```python
from build123d import *

# Parameters (mm, degrees)
F0_W     = 30
F0_H     = 30
F1_DEPTH = 10
F3_DEPTH = 25


with BuildPart() as f1:
    # F0 (on Front) → F1 (new body)
    with BuildSketch(Plane.XZ):
        with Locations((15, -15)):
            Rectangle(F0_W, F0_H)
    extrude(amount=F1_DEPTH)

    # F2 (on face) → F3 (cut)
    with BuildSketch(Plane.XZ.offset(10)):
        with BuildLine():
            ThreePointArc((5.35, -25), (4, -23.65), (2.65, -25))
            Line((2.65, -25), (5.35, -25))
        make_face()
        with BuildLine():
            Line((5.35, -25), (2.65, -25))
            ThreePointArc((2.65, -25), (4, -26.35), (5.35, -25))
        make_face()
        with BuildLine():
            ThreePointArc((27.35, -25), (26, -23.65), (24.65, -25))
            Line((24.65, -25), (27.35, -25))
        make_face()
        with BuildLine():
            Line((27.35, -25), (24.65, -25))
            ThreePointArc((24.65, -25), (26, -26.35), (27.35, -25))
        make_face()
        with BuildLine():
            Line((27.35, -5), (24.65, -5))
            ThreePointArc((24.65, -5), (26, -6.35), (27.35, -5))
        make_face()
        with BuildLine():
            ThreePointArc((27.35, -5), (26, -3.65), (24.65, -5))
            Line((24.65, -5), (27.35, -5))
        make_face()
        with BuildLine():
            Line((5.35, -5), (2.65, -5))
            ThreePointArc((2.65, -5), (4, -6.35), (5.35, -5))
        make_face()
        with BuildLine():
            ThreePointArc((5.35, -5), (4, -3.65), (2.65, -5))
            Line((2.65, -5), (5.35, -5))
        make_face()
    extrude(amount=-F3_DEPTH, mode=Mode.SUBTRACT)


solid = f1.part
```
Work out the finished part from the listing and answer in its coordinate system (mm). Give positions to 0.01 mm unless a question says otherwise; leave off trailing zeros. Order: outer loops, then holes, each group sorted by start corner. A loop starts at its lowest first (then second) coordinate and runs counter-clockwise, first axis right, second up. Notation, with made-up numbers: (73.25, 79) -> (132.25, 79) arc R9 ccw to (132.25, 86) -> close; hole circle Ø7 at (76, 49). An arc over 180 degrees is marked (long way). Answer as CSV lines item,"result". Start each with the question number.
(1) Section B-B, the plane y = -4 is taken. Write down the section's boundary in (x, z), plus the area to 3 significant figures.
(2) Consider line 1 along Z through (x, y) = (4, -5.5); line 2 along X through (y, z) = (-3.25, -25). Determine where each line is inside the solid, lowest interval first.
(3) Section A-A, the plane x = 26 is taken. Write down the section's boundary in (y, z), plus the area to 3 significant figures.
(4) Section C-C, the plane z = -5 is taken. Write down the section's boundary in (x, y), plus the area to 3 significant figures.
(5) For a pull along Z with two mould halves and no side action, classify faces 1 (the flat face through (15, -5, 0)), 2 (the flat face through (15, -10, -15)), 3 (the flat face through (15, -5, -30)), 4 (the cylindrical face through (27.247, -5.07, -5.517)) as released by +Z, released by -Z, zero draft, split by the parting line, or undercut.
(6) This flat-tipped pin is pushed along its axis until it touches: pin 1 Ø2 at (x, z) = (4, -5) entering from +Y. Where does it stop, or does it pass through?
Entries:
1,outline,"(0, -30) -> (30, -30) -> (30, 0) -> (0, 0) -> close; hole circle Ø2.7 at (4, -25); hole circle Ø2.7 at (4, -5); hole circle Ø2.7 at (26, -25); hole circle Ø2.7 at (26, -5)"
1,area,"877 mm²"
2,line 1,"-30 to -26.35, -23.65 to -6.35, -3.65 to 0"
2,line 2,"0 to 2.65, 5.35 to 24.65, 27.35 to 30"
3,outline,"(-10, -30) -> (0, -30) -> (0, -26.35) -> (-10, -26.35) -> close; (-10, -23.65) -> (0, -23.65) -> (0, -6.35) -> (-10, -6.35) -> close; (-10, -3.65) -> (0, -3.65) -> (0, 0) -> (-10, 0) -> close"
3,area,"246 mm²"
4,outline,"(0, -10) -> (2.65, -10) -> (2.65, 0) -> (0, 0) -> close; (5.35, -10) -> (24.65, -10) -> (24.65, 0) -> (5.35, 0) -> close; (27.35, -10) -> (30, -10) -> (30, 0) -> (27.35, 0) -> close"
4,area,"246 mm²"
5,face 1,"released by +Z"
5,face 2,"zero draft"
5,face 3,"released by -Z"
5,face 4,"undercut"
6,pin 1,"through"
